Autodesk Inventor part; units mm, degrees
ref_plane "YZ Plane" through (0, 0, 0) normal (1, 0, 0) x (0, 1, 0)
ref_plane "XZ Plane" through (0, 0, 0) normal (0, 1, 0) x (-1, 0, 0)
ref_plane "XY Plane" through (0, 0, 0) normal (0, 0, 1) x (1, 0, 0)
sketch "Sketch2" plane through (0, 0, 0) normal (0, 1, 0) x (-1, 0, 0)
  circle A0 centre (0, 0) radius 3.52 construction
  circle A1 centre (0, 0) radius 2.3784 construction
  line L0 (-4, 4) -> (4, 4) construction
  line L1 (4, 4) -> (4, -4) construction
  line L2 (-0.8, 2.2399) -> (-0.8, 0.8)
  line L3 (-0.8, 0.8) -> (-2.2399, 0.8)
  line L4 (-2.2399, -0.8) -> (-0.8, -0.8)
  line L5 (-0.8, -0.8) -> (-0.8, -2.2399)
  line L6 (0.8, -2.2399) -> (0.8, -0.8)
  line L7 (0.8, -0.8) -> (2.2399, -0.8)
  line L8 (2.2399, 0.8) -> (0.8, 0.8)
  line L9 (0.8, 0.8) -> (0.8, 2.2399)
  arc A2 (0.8, 2.2399) -> (-0.8, 2.2399) centre (0, 0) ccw
  arc A3 (-2.2399, 0.8) -> (-2.2399, -0.8) centre (0, 0) ccw
  arc A4 (-0.8, -2.2399) -> (0.8, -2.2399) centre (0, 0) ccw
  arc A5 (2.2399, -0.8) -> (2.2399, 0.8) centre (0, 0) ccw
  circle A6 centre (-4, 4) radius 2.4
  circle A7 centre (4, 4) radius 2.4
  circle A8 centre (-4, -4) radius 2.4
  circle A9 centre (4, -4) radius 2.4
  arc A10 (1.6845, 3.3686) -> (-1.6845, 3.3686) centre (0, -5.93) ccw
  line L10 (-3.4, 1.6762) -> (-3.4, -1.6762)
  line L11 (3.4, 1.6762) -> (3.4, -1.6762)
  arc A11 (-1.6845, -3.3686) -> (1.6845, -3.3686) centre (0, 5.93) ccw
  circle A12 centre (0, 0) radius 1.1314
  point P0 (0, 4)
  point P1 (4, 0)
  dimension "d0" = 4.7569
  dimension "d1" = 7.04
  dimension "d2" = 8
  dimension "d4" = 1.6
  dimension "d20" = 4.8
  dimension "d21" = 18.9
  dimension "d22" = 6.8
extrude "Extrusion1" add sketch "Sketch2" along normal mid plane 16 contours A6 A10 A7 L11 A9 A11 A8 L10
extrude "Extrusion3" add sketch "Sketch2" along normal mid plane 0.2 contours A2 L9 A12 L2 | A12 L4 A3 L3 | L8 A5 L7 A12 | A12 L6 A4 L5
fillet "Fillet1" radius 0.1 8 edges at (1.6845, 0, 3.3686) (3.4, 0, 1.6762) (-1.6845, 0, 3.3686) (-3.4, 0, 1.6762) (3.4, 0, -1.6762) (1.6845, 0, -3.3686) (-1.6845, 0, -3.3686) (-3.4, 0, -1.6762)
equation "\"d2\" = lu"
equation "\"d4\" = axlet"
properties part number "6538c-Black" material "ABS Plastic"
Source: CAD feature listing. Evaluate the final solid. Frame: model axes, mm. A direction names the side the tool comes from. Give positions to 0.01 mm unless a question says otherwise; leave off trailing zeros. Write each loop counter-clockwise with the first axis right and the second up, starting at its lowest first coordinate (ties: lowest second). Pieces come first, ordered by that corner, then holes. Notation, with made-up numbers: M 18,-3.5 L 34,-3.5 A30 ccw 34,19.5 Z; hole C -15,-25 d1. An arc over 180 degrees is marked long. Return JSON: item names as keys, results as strings. Group by question number.
1) Set-up query: faces 1 (the face through (-2.322, -0.112, 2.285)), 2 (the face through (0.8, 4, 2)), 3 (the face through (2, -0.1, 0)). Return all of +Z, -Z, +X, -X, +Y, -Y with unobstructed straight access to the full face (end or side cutting, diameter ignored); none if empty.
2) Cut plane A-A, the plane x = 0. Output: boundary loops of the cut face in (y, z), plus the area to 3 significant figures.
3) Cut plane B-B, the plane z = 0. Output: boundary loops of the cut face in (x, y).
4) Pull-direction query (Z, two-part tool) for faces 4 (the face through (-0.8, 4, 2)), 5 (the face through (2.322, -0.112, -2.285)), 6 (the face through (-2.38, -4.11, 0.01)), 7 (the face through (-3.4, 0, 0)); classes: pulls with the +Z half, pulls with the -Z half, needs draft (parallel to the pull), parting line crosses it, or undercut.
5) Pin query (flat end, axial travel): P1, Ø1, axis at y = 5.5, z = -2.5, coming from the -X side; P2, Ø1, axis at x = -1.5, y = 3, coming from the +Z side; P3, Ø1, axis at x = -2.5, y = -4, coming from the +Z side. Return the tip coordinate at first contact, or that it passes through.
6) Material intervals for line 1 along X through (y, z) = (0, 0); line 2 along Z through (x, y) = (-1.5, 2.5), sorted ascending. Write a range as [from, to].
Recorded:
{
 "1": {"face 1": "+Z, -X, +Y, -Y", "face 2": "+Y", "face 3": "-Y"},
 "2": {"outline": "M -8,-3.52 L 8,-3.52 L 8,-2.38 L 0.1,-2.38 L 0.1,-1.13 L -0.1,-1.13 L -0.1,-2.38 L -8,-2.38 Z; M -8,2.38 L -0.1,2.38 L -0.1,1.13 L 0.1,1.13 L 0.1,2.38 L 8,2.38 L 8,3.52 L -8,3.52 Z", "area": "37.0 mm²"},
 "3": {"outline": "M -3.4,-8 L -2.38,-8 L -2.38,-0.1 L -1.13,-0.1 L -1.13,0.1 L -2.38,0.1 L -2.38,8 L -3.4,8 Z; M 1.13,-0.1 L 2.38,-0.1 L 2.38,-8 L 3.4,-8 L 3.4,8 L 2.38,8 L 2.38,0.1 L 1.13,0.1 Z"},
 "4": {"face 4": "undercut", "face 5": "pulls with the -Z half", "face 6": "undercut", "face 7": "needs draft"},
 "5": {"P1": "stops at x = -2.67", "P2": "stops at z = 3.47", "P3": "stops at z = 2.67"},
 "6": {"line 1": "x = [-3.4, -1.13], [1.13, 3.4]", "line 2": "z = [-3.4, -0.8], [0.8, 3.4]"}
}
